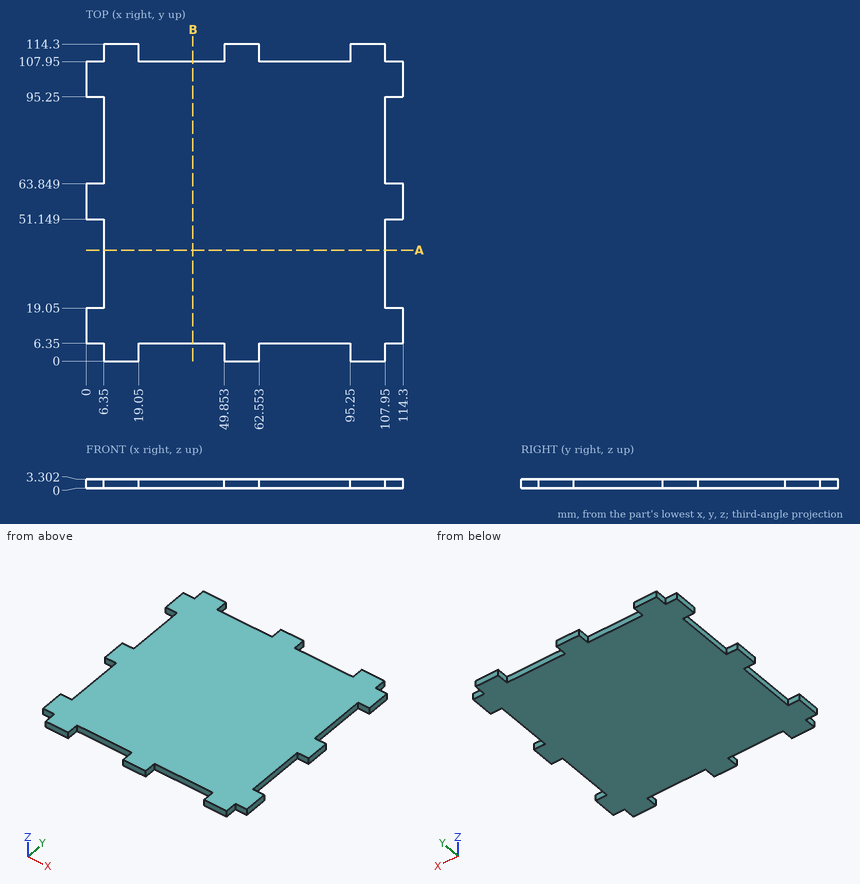
Check sheet for the drawn part. Datum: minimum x, y, z corner. Units: mm. Coordinates: 2 decimals unless noted, no trailing zeros. Order: outer loops, then holes, each group sorted by start corner. A loop starts at its lowest first (then second) coordinate and runs counter-clockwise, first axis right, second up. Notation, with made-up numbers: (-1, -29) - (53, -29) arc R30 ccw to (53, 1) - close; hole circle Ø7 at (-17.75, -28). An arc over 180 degrees is marked (long way). Return JSON: item names as keys, results as strings.
(1) Thickness scan on line 1 along Y through (x, z) = (110.5, 2); line 2 along X through (y, z) = (66.5, 1.2). Record the ranges inside material, lowest first.
Filled sheet:
{"line 1": "y = 6.35 to 19.05, 51.15 to 63.85, 95.25 to 107.95", "line 2": "x = 6.35 to 107.95"}
(2) Go/stop test with flat-tipped pins: pin 1 (1.7 mm diameter, centred on x = 3.5, z = 1.5, fed in from -Y); pin 2 (1.7 mm diameter, centred on y = 112.5, z = 1, fed in from +X); pin 3 (1.7 mm diameter, centred on y = 111.5, z = 1.5, fed in from -X). Record where each tip stops, or that it passes through.
Filled sheet:
{"pin 1": "stops at y = 6.35", "pin 2": "stops at x = 107.95", "pin 3": "stops at x = 6.35"}
(3) Section check A-A, the plane y = 40. Record the cut outline in (x, z).
Filled sheet:
{"outline": "(6.35, 0) - (107.95, 0) - (107.95, 3.3) - (6.35, 3.3) - close"}
